from build123d import *

# Parameters (mm, degrees)
SKETCH1_W           = 30
SKETCH1_H           = 60.05
BOSS_EXTRUDE1_DEPTH = 3.15
CUT_EXTRUDE1_DEPTH  = 3.15
SKETCH3_R           = 1.3
CUT_EXTRUDE2_DEPTH  = 3.15
FILLET1_R           = 1.5
SKETCH5_R           = 1.3
CUT_EXTRUDE3_DEPTH  = 3.15


with BuildPart() as part:
    # Sketch1 → Boss-Extrude1 (new body)
    with BuildSketch(Plane(origin=(0, 0, 0), x_dir=(1, 0, 0), z_dir=(0, 1, 0))):
        Rectangle(SKETCH1_W, SKETCH1_H)
    extrude(amount=-BOSS_EXTRUDE1_DEPTH)

    # Sketch2 → Cut-Extrude1 (cut)
    with BuildSketch(Plane(origin=(0, 0, 0), x_dir=(1, 0, 0), z_dir=(0, 1, 0))):
        with BuildLine():
            Line((-8.5, 13.975), (8.5, 13.975))
            ThreePointArc((8.5, 13.975), (9.560660172, 13.535660172), (10, 12.475))
            Line((10, 12.475), (10, 5.475))
            ThreePointArc((10, 5.475), (9.560660172, 4.414339828), (8.5, 3.975))
            Line((8.5, 3.975), (-8.5, 3.975))
            ThreePointArc((-8.5, 3.975), (-9.560660172, 4.414339828), (-10, 5.475))
            Line((-10, 5.475), (-10, 12.475))
            ThreePointArc((-10, 12.475), (-9.560660172, 13.535660172), (-8.5, 13.975))
        make_face()
        with BuildLine():
            Line((-8.5, -8.025), (8.5, -8.025))
            ThreePointArc((8.5, -8.025), (9.560660172, -8.464339828), (10, -9.525))
            Line((10, -9.525), (10, -16.525))
            ThreePointArc((10, -16.525), (9.560660172, -17.585660172), (8.5, -18.025))
            Line((8.5, -18.025), (-8.5, -18.025))
            ThreePointArc((-8.5, -18.025), (-9.560660172, -17.585660172), (-10, -16.525))
            Line((-10, -16.525), (-10, -9.525))
            ThreePointArc((-10, -9.525), (-9.560660172, -8.464339828), (-8.5, -8.025))
        make_face()
    extrude(amount=-CUT_EXTRUDE1_DEPTH, mode=Mode.SUBTRACT)

    # Sketch3 → Cut-Extrude2 (cut)
    with BuildSketch(Plane(origin=(0, 0, 0), x_dir=(1, 0, 0), z_dir=(0, 1, 0))):
        with Locations((-11, 27.425)):
            Circle(SKETCH3_R)
        with Locations((11, 27.425)):
            Circle(SKETCH3_R)
    extrude(amount=-CUT_EXTRUDE2_DEPTH, mode=Mode.SUBTRACT)

    # Fillet1
    fillet1_edges = [part.edges().sort_by_distance(p)[0] for p in [
        (-15, -1.575, -30.025),
        (15, -1.575, -30.025),
        (15, -1.575, 30.025),
        (-15, -1.575, 30.025),
    ]]
    fillet(fillet1_edges, radius=FILLET1_R)

    # Sketch5 → Cut-Extrude3 (cut)
    with BuildSketch(Plane(origin=(0, 0, 0), x_dir=(1, 0, 0), z_dir=(0, 1, 0))):
        with Locations((-7.75, -2.025)):
            Circle(SKETCH5_R)
        with Locations((7.75, -2.025)):
            Circle(SKETCH5_R)
        with Locations((-7.75, -21.65)):
            Circle(SKETCH5_R)
        with Locations((7.75, -21.65)):
            Circle(SKETCH5_R)
    extrude(amount=-CUT_EXTRUDE3_DEPTH, mode=Mode.SUBTRACT)


solid = part.part
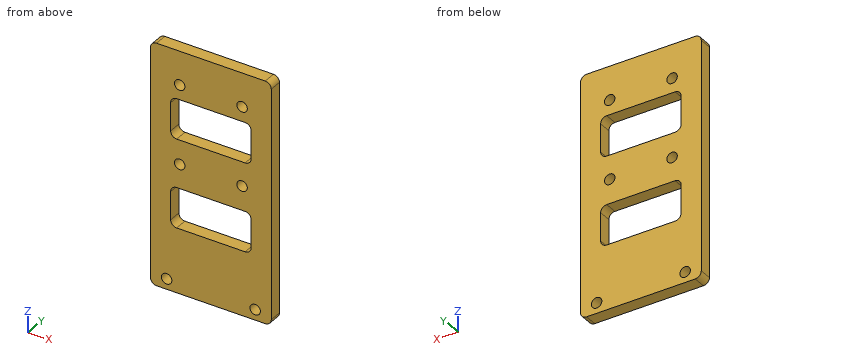
Geometry: final body of the model. Coordinates: model frame, mm. Give positions to 0.01 mm unless a question says otherwise; leave off trailing zeros. Write each loop counter-clockwise with the first axis right and the second up, starting at its lowest first coordinate (ties: lowest second). Pieces come first, ordered by that corner, then holes.
(1) Cut plane D-D, the plane y = -2.1. Give the number of separate pieces and of enclosed holes in the cut face, then the cut area to 3 significant figures.
(2) Ray query, line 1 (Z direction, x = -7.75, y = -2) (3 decimals); line 2 (Z direction, x = -2.75, y = -1.8) (3 decimals); line 3 (X direction, y = -1.8, z = 21.65). Return the intervals inside material, ascending.
(3) Cut plane B-B, the plane x = 11. Return loops of the section in (y, z) (3 decimals), then the cut area to 3 significant figures.
(4) Cut plane C-C, the plane z = 10.5. Return loops of the section in (x, y).
(5) Cut plane A-A, the plane z = 21.65. Return loops of the section in (x, y).
Values follow:
1. separate pieces: 1
1. enclosed holes: 8
1. area: 1,370 mm2
2. line 1: z = -30.025 to -13.975, -3.975 to 0.725, 3.325 to 8.025, 18.025 to 20.35, 22.95 to 30.025
2. line 2: z = -30.025 to -13.975, -3.975 to 8.025, 18.025 to 30.025
2. line 3: x = -15 to -9.05, -6.45 to 6.45, 9.05 to 15
3. outline: (-3.15, -30.025) - (0, -30.025) - (0, -28.725) - (-3.15, -28.725) - close; (-3.15, -26.125) - (0, -26.125) - (0, 30.025) - (-3.15, 30.025) - close
3. area: 181 mm2
4. outline: (-15, -3.15) - (-10, -3.15) - (-10, 0) - (-15, 0) - close; (10, -3.15) - (15, -3.15) - (15, 0) - (10, 0) - close
5. outline: (-15, -3.15) - (-9.05, -3.15) - (-9.05, 0) - (-15, 0) - close; (-6.45, -3.15) - (6.45, -3.15) - (6.45, 0) - (-6.45, 0) - close; (9.05, -3.15) - (15, -3.15) - (15, 0) - (9.05, 0) - close
